Source: CAD feature listing. Evaluate the final solid. Frame: model axes, mm. A direction names the side the tool comes from. Give positions to 0.01 mm unless a question says otherwise; leave off trailing zeros. Loops run counter-clockwise (first coordinate to the right, second up) from the corner with the lowest first, then second, coordinate; pieces in that order, holes last. Notation, with made-up numbers: (-24, 52) -> (-7, 52) arc R23 ccw to (-7, 81) -> close; hole circle Ø3 at (-5, 65.25). An arc over 180 degrees is marked (long way). Put each result on its own line as item: value.
```python
from build123d import *

# Parameters (mm, degrees)
F0_R     = 1.5
F1_DEPTH = 1.3


with BuildPart() as f1:
    # F0 (on Front) → F1 (new body)
    with BuildSketch(Plane.XZ):
        with BuildLine():
            ThreePointArc((-8.391363, -5.463446), (-9.461447, -6.161412), (-10.673479, -6.565408))
            ThreePointArc((-10.673479, -6.565408), (-12.474874, -12.474874), (-6.565408, -10.673479))
            ThreePointArc((-6.565408, -10.673479), (-6.161412, -9.461447), (-5.463446, -8.391363))
            ThreePointArc((-5.463446, -8.391363), (0, -5.870058), (5.463446, -8.391363))
            ThreePointArc((5.463446, -8.391363), (6.161412, -9.461447), (6.565408, -10.673479))
            ThreePointArc((6.565408, -10.673479), (12.474874, -12.474874), (10.673479, -6.565408))
            ThreePointArc((10.673479, -6.565408), (9.461447, -6.161412), (8.391363, -5.463446))
            ThreePointArc((8.391363, -5.463446), (5.870058, 0), (8.391363, 5.463446))
            ThreePointArc((8.391363, 5.463446), (9.461447, 6.161412), (10.673479, 6.565408))
            ThreePointArc((10.673479, 6.565408), (12.474874, 12.474874), (6.565408, 10.673479))
            ThreePointArc((6.565408, 10.673479), (6.161412, 9.461447), (5.463446, 8.391363))
            ThreePointArc((5.463446, 8.391363), (0, 5.870058), (-5.463446, 8.391363))
            ThreePointArc((-5.463446, 8.391363), (-6.161412, 9.461447), (-6.565408, 10.673479))
            ThreePointArc((-6.565408, 10.673479), (-12.474874, 12.474874), (-10.673479, 6.565408))
            ThreePointArc((-10.673479, 6.565408), (-9.461447, 6.161412), (-8.391363, 5.463446))
            ThreePointArc((-8.391363, 5.463446), (-5.870058, 0), (-8.391363, -5.463446))
        make_face()
        with Locations((-10, -10)):
            Circle(F0_R, mode=Mode.SUBTRACT)
        with Locations((10, -10)):
            Circle(F0_R, mode=Mode.SUBTRACT)
        with Locations((-10, 10)):
            Circle(F0_R, mode=Mode.SUBTRACT)
        with Locations((10, 10)):
            Circle(F0_R, mode=Mode.SUBTRACT)
    extrude(amount=F1_DEPTH)


solid = f1.part
```
(1) Line query: probe 1 along Z at (x, y) = (11, -0.75); probe 2 along Z at (x, y) = (-10, -0.85); probe 3 along Z at (x, y) = (-7.5, -0.1). Output: solid intervals per line, ascending. Write a range as from..to.
Calculated:
probe 1: z = -13.35..-11.12, -8.88..-6.65, 6.65..8.88, 11.12..13.35
probe 2: z = -13.5..-11.5, -8.5..-6.38, 6.38..8.5, 11.5..13.5
probe 3: z = -12.45..-4.56, 4.56..12.45
(2) Section D-D on x = -10. Return loops of the section in (y, z), then the cut area to 3 significant figures.
Calculated:
outline: (-1.3, -13.5) -> (0, -13.5) -> (0, -11.5) -> (-1.3, -11.5) -> close; (-1.3, -8.5) -> (0, -8.5) -> (0, -6.38) -> (-1.3, -6.38) -> close; (-1.3, 6.38) -> (0, 6.38) -> (0, 8.5) -> (-1.3, 8.5) -> close; (-1.3, 11.5) -> (0, 11.5) -> (0, 13.5) -> (-1.3, 13.5) -> close
area: 10.7 mm²
(3) Section C-C on z = -10. Return loops of the section in (x, y), then the cut area to 3 significant figures.
Calculated:
outline: (-13.5, -1.3) -> (-11.5, -1.3) -> (-11.5, 0) -> (-13.5, 0) -> close; (-8.5, -1.3) -> (-6.38, -1.3) -> (-6.38, 0) -> (-8.5, 0) -> close; (6.38, -1.3) -> (8.5, -1.3) -> (8.5, 0) -> (6.38, 0) -> close; (11.5, -1.3) -> (13.5, -1.3) -> (13.5, 0) -> (11.5, 0) -> close
area: 10.7 mm²
(4) Draft query along Z for faces 1 (the flat face through (0, 0, 0)), 2 (the cylindrical face through (-6.17, -0.64, -9.48)), 3 (the cylindrical face through (5.87, -0.64, -0.09)), 4 (the cylindrical face through (-12.4, -0.64, 12.55)). Return one class per face: released by +Z, released by -Z, zero draft, split by the parting line, or undercut.
Calculated:
face 1: zero draft
face 2: released by -Z
face 3: undercut
face 4: undercut
(5) Reachability of faces 5 (the cylindrical face through (-9.445, -0.641, -6.154)), 6 (the cylindrical face through (6.17, -0.64, 9.48)), 7 (the cylindrical face through (9.445, -0.641, 6.154)) from +Z, -Z, +X, -X, +Y, -Y: full face, straight path, thin tool, end or side. Return the list, or none.
Calculated:
face 5: -X, +Y, -Y
face 6: +Z, +Y, -Y
face 7: +X, +Y, -Y
(6) Section B-B on y = -0.35. Return loops of the section in (x, z).
Calculated:
outline: (-10.67, -6.57) arc R3.5 ccw (long way) to (-6.57, -10.67) arc R5 cw to (-5.46, -8.39) arc R7.18 cw to (5.46, -8.39) arc R5 cw to (6.57, -10.67) arc R3.5 ccw (long way) to (10.67, -6.57) arc R5 cw to (8.39, -5.46) arc R7.18 cw to (8.39, 5.46) arc R5 cw to (10.67, 6.57) arc R3.5 ccw (long way) to (6.57, 10.67) arc R5 cw to (5.46, 8.39) arc R7.18 cw to (-5.46, 8.39) arc R5 cw to (-6.57, 10.67) arc R3.5 ccw (long way) to (-10.67, 6.57) arc R5 cw to (-8.39, 5.46) arc R7.18 cw to (-8.39, -5.46) arc R5 cw to start; hole circle Ø3 at (-10, -10); hole circle Ø3 at (-10, 10); hole circle Ø3 at (10, -10); hole circle Ø3 at (10, 10)
(7) Section A-A on x = 7.75. Return loops of the section in (y, z).
Calculated:
outline: (-1.3, -12.68) -> (0, -12.68) -> (0, -4.84) -> (-1.3, -4.84) -> close; (-1.3, 4.84) -> (0, 4.84) -> (0, 12.68) -> (-1.3, 12.68) -> close
